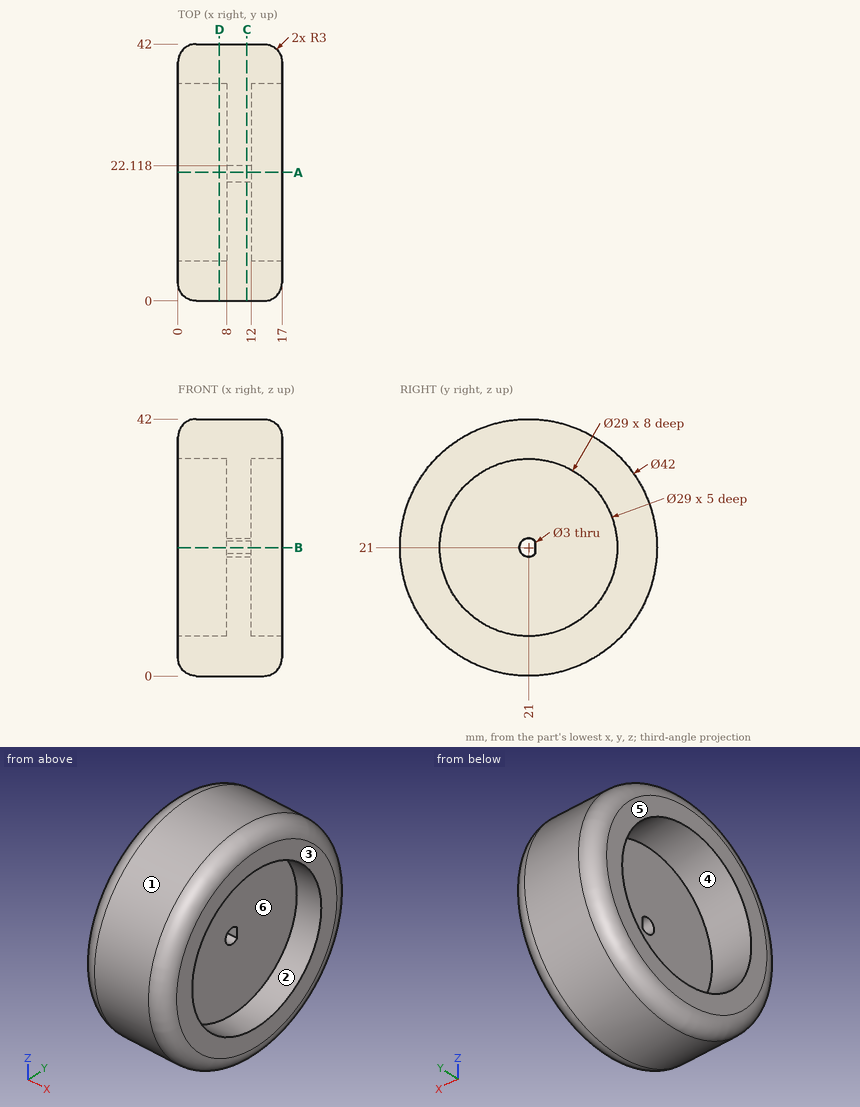
Can you work these out from the drawing? Everything is in mm from the part's minimum corner. A direction names the side the tool comes from. Give positions to 0.01 mm unless a question says otherwise; leave off trailing zeros. Order: outer loops, then holes, each group sorted by start corner. A loop starts at its lowest first (then second) coordinate and runs counter-clockwise, first axis right, second up. Notation, with made-up numbers: M 14.25,-23.5 L 66.25,-23.5 A25 cw 66.25,0.5 Z; hole C 40,-30 d9. An arc over 180 degrees is marked long. Use a Markdown table: item, result. Add a question column.
1. I need wall thicknesses on probe 1 along Y at (x, z) = (13.2, 21); probe 2 along Y at (x, z) = (15.2, 21); probe 3 along Z at (x, y) = (5, 11.5). Which ranges of each line are inside material? Lowest first, please. Write a range as from..to.
2. On a 3-axis mill with a long thin cutter (end or side, diameter ignored), from which of +Z, -Z, +X, -X, +Y, -Y can I reach the whole of each face in a straight line? I mean the marked faces 4, 5 and 6. Say none if no direction works.
3. If we mould it in two halves opening along Y, with no side actions, what happens to the marked faces 1, 2 and 3? For each: +Y half, -Y half, draft (parallel to the pull), parting line (faces both ways), or undercut.
4. Suppose I cut it at C-C (x = 11.25). List the corners of the cut face in (y, z) for me, and give its area (3 significant figures).
5. Suppose I cut it at A-A (y = 21). List the corners of the cut face in (x, z) for me.
6. Suppose I cut it at D-D (x = 6.75). List the corners of the cut face in (y, z) for me.
7. For pin 1 Ø5 at (x, y) = (7, 4.5) entering from -Z; pin 2 Ø5 at (x, y) = (5.5, 22.5) entering from -Z; pin 3 Ø1 at (x, y) = (11.5, 9) entering from -Z; pin 4 Ø8 at (x, z) = (15, 22.5) entering from +Y, each with a flat end and sliding along its axis, tell me the tip position at first contact or that it passes through.
8. Suppose I cut it at B-B (z = 21). List the corners of the cut face in (x, y) for me, and give its area (3 significant figures).
Results list:
| question | item | result |
|---|---|---|
| 1 | probe 1 | y = 0..6.5, 35.5..42 |
| 1 | probe 2 | y = 0.25..6.5, 35.5..41.75 |
| 1 | probe 3 | z = 2.27..10.05, 31.95..39.73 |
| 2 | face 4 | -X |
| 2 | face 5 | +Z, -Z, -X, +Y, -Y |
| 2 | face 6 | +X |
| 3 | face 1 | parting line |
| 3 | face 2 | undercut |
| 3 | face 3 | draft |
| 4 | outline | C 21,21 d42; hole M 22.12,20 L 22.12,22 A1.5 ccw long Z |
| 4 | area | 1,380 mm² |
| 5 | outline | M 0,3 A3 ccw 3,0 L 14,0 A3 ccw 17,3 L 17,6.5 L 12,6.5 L 12,19.5 L 8,19.5 L 8,6.5 L 0,6.5 Z; M 0,35.5 L 8,35.5 L 8,22.5 L 12,22.5 L 12,35.5 L 17,35.5 L 17,39 A3 ccw 14,42 L 3,42 A3 ccw 0,39 Z |
| 6 | outline | C 21,21 d42; hole C 21,21 d29 |
| 7 | pin 1 | stops at z = 5.35 |
| 7 | pin 2 | stops at z = 0 |
| 7 | pin 3 | stops at z = 3.43 |
| 7 | pin 4 | stops at y = 42 |
| 8 | outline | M 0,3 A3 ccw 3,0 L 14,0 A3 ccw 17,3 L 17,6.5 L 12,6.5 L 12,19.5 L 8,19.5 L 8,6.5 L 0,6.5 Z; M 0,35.5 L 8,35.5 L 8,22.12 L 12,22.12 L 12,35.5 L 17,35.5 L 17,39 A3 ccw 14,42 L 3,42 A3 ccw 0,39 Z |
| 8 | area | 319 mm² |
